For this review, take the finished solid that the model builds, in its own axes (mm). Coordinates: 2 decimals unless noted, no trailing zeros. Order: outer loops, then holes, each group sorted by start corner. A loop starts at its lowest first (then second) coordinate and runs counter-clockwise, first axis right, second up. Notation, with made-up numbers: (-35, 7.25) -> (-5, 7.25) arc R19 ccw to (-5, 40.25) -> close; hole circle Ø2 at (-21, 45.5). An arc over 180 degrees is marked (long way). Write item = value, one per line. Start each with the question number.
1) Consider section B-B on y = -4.75. Give the boundary of the cut face in (x, z), and give its area (3 significant figures).
2) Consider section C-C on z = 1.5. Give the boundary of the cut face in (x, y).
3) Insertion check: pin 1 Ø1.8 at (x, y) = (-27.89, -5.46) entering from +Z. The pin has a flat end and moves straight along its axis. Give the tip position at first contact, or say it passes through.
4) Wall thickness on probe 1 along X at (y, z) = (13.25, 0.3); probe 2 along X at (y, z) = (11, 0.95); probe 3 along Y at (x, z) = (-37, 0.6): over which ranges is each line inside the solid? List them lowest first. Write a range as [from, to].
5) Consider section A-A on x = -18.75. Give the boundary of the cut face in (y, z).
6) Draft analysis for pull direction X (two halves, no side actions). For faces 1 (the face through (-26.457, -5.013, 0.986)), 2 (the face through (-40.887, 1, 1)), 3 (the face through (-28, 2, 0)), state which applies: +X half, -X half, draft (parallel to the pull), parting line (faces both ways), or undercut.
from build123d import *

# Parameters (mm, degrees)
CROQUIS1_W              = 26
CROQUIS1_H              = 28
CROQUIS1_R              = 1.5
SALIENTE_EXTRUIR1_DEPTH = 2


with BuildPart() as part:
    # Croquis1 → Saliente-Extruir1 (new body)
    with BuildSketch(Plane.XY):
        with Locations((-27.887270297, 1.536585366)):
            Rectangle(CROQUIS1_W, CROQUIS1_H)
        with Locations((-37.387270297, 12.036585366)):
            Circle(CROQUIS1_R, mode=Mode.SUBTRACT)
        with Locations(Location((-18.387270297, 12.036585366, 0), (0, 0, 180))):
            Circle(CROQUIS1_R, mode=Mode.SUBTRACT)
        with Locations((-27.887270297, -5.463414634)):
            Circle(CROQUIS1_R, mode=Mode.SUBTRACT)
    extrude(amount=SALIENTE_EXTRUIR1_DEPTH)


solid = part.part
Answer sheet:
q1.outline = (-40.89, 0) -> (-29.21, 0) -> (-29.21, 2) -> (-40.89, 2) -> close; (-26.57, 0) -> (-14.89, 0) -> (-14.89, 2) -> (-26.57, 2) -> close
q1.area = 46.7 mm2
q2.outline = (-40.89, -12.46) -> (-14.89, -12.46) -> (-14.89, 15.54) -> (-40.89, 15.54) -> close; hole circle Ø3 at (-37.39, 12.04); hole circle Ø3 at (-27.89, -5.46); hole circle Ø3 at (-18.39, 12.04)
q3.pin_1 = through
q4.probe_1 = [-40.89, -38.27], [-36.51, -19.27], [-17.51, -14.89]
q4.probe_2 = [-40.89, -38.47], [-36.3, -19.47], [-17.3, -14.89]
q4.probe_3 = [-12.46, 10.59], [13.49, 15.54]
q5.outline = (-12.46, 0) -> (10.58, 0) -> (10.58, 2) -> (-12.46, 2) -> close; (13.49, 0) -> (15.54, 0) -> (15.54, 2) -> (13.49, 2) -> close
q6.face_1 = undercut
q6.face_2 = -X half
q6.face_3 = draft
